The listing builds one solid part. Answer for the finished solid, in the listing's coordinates (mm). Give positions to 0.01 mm unless a question says otherwise; leave off trailing zeros. Order: outer loops, then holes, each group sorted by start corner. A loop starts at its lowest first (then second) coordinate and runs counter-clockwise, first axis right, second up.
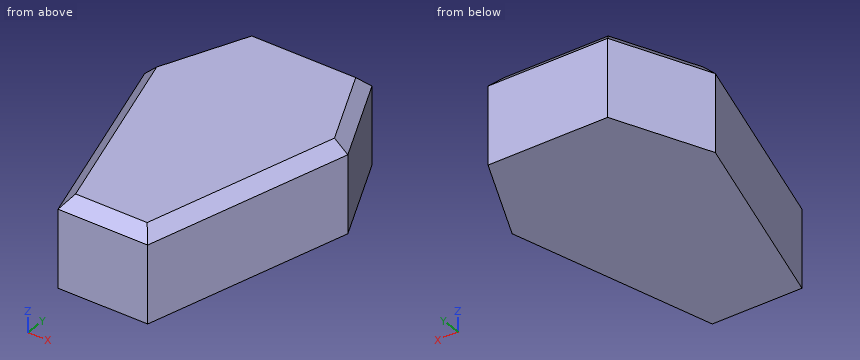
```python
from build123d import *

# Parameters (mm, degrees)
F1_DEPTH = 38.1
F2_SIZE  = 5.08
F3_T     = -7.62


with BuildPart() as f1:
    # F0 (on Top) → F1 (new body)
    with BuildSketch(Plane.XY):
        Polygon((17.9854446539, 64.1556447676), (-32.8145553461, 64.1556447676), (-50.5846425152, 24.8016563801), (-26.4645553461, -60.7637069099), (11.6354446539, -60.7637069099), (35.7555318229, 24.8016563801), align=None)
    extrude(amount=F1_DEPTH)

    # F2
    f2_edges = [f1.edges().sort_by_distance(p)[0] for p in [
        (-41.699599, 44.478651, 38.1),
        (-7.414555, 64.155645, 38.1),
        (26.870488, 44.478651, 38.1),
        (23.695488, -17.981025, 38.1),
        (-38.524599, -17.981025, 38.1),
        (-7.414555, -60.763707, 38.1),
    ]]
    chamfer(f2_edges, length=F2_SIZE)

    # F3 (hollow: no face is removed)
    offset(amount=F3_T, kind=Kind.INTERSECTION, mode=Mode.SUBTRACT)


solid = f1.part
```
1) Straight lines are drawn through the part: probe 1 along Z at (x, y) = (10, 4.5); probe 2 along Y at (x, z) = (-17, 24); probe 3 along X at (y, z) = (-48, 21.5). For each, find the intervals that lie inside material, in ascending order.
Geometry says:
probe 1: z = 0 to 7.62, 30.48 to 38.1
probe 2: y = -60.76 to -53.14, 56.54 to 64.16
probe 3: x = -30.06 to -22.15, 7.32 to 15.23
2) Find section A-A (x = -13). Write down the section's boundary in (y, z), then the cut area to 3 significant figures.
Geometry says:
outline: (-60.76, 0) - (64.16, 0) - (64.16, 33.02) - (59.08, 38.1) - (-55.68, 38.1) - (-60.76, 33.02) - close; hole (-53.14, 7.62) - (56.54, 7.62) - (56.54, 29.86) - (55.92, 30.48) - (-52.53, 30.48) - (-53.14, 29.86) - close
area: 2,230 mm2
3) Given P1, Ø10, axis at y = 2, z = 25.5, coming from the +X side; P2, Ø12, axis at y = -36, z = 26, coming from the -X side; P3, Ø10, axis at y = 15.5, z = 12.5, coming from the +X side, each flat-ended and moving along its own axis, determine where each tip first touches the part or whether it passes through.
Geometry says:
P1: stops at x = 30.74
P2: stops at x = -35.14
P3: stops at x = 34.54
4) Find section B-B (z = 22). Write down the section's boundary in (x, y).
Geometry says:
outline: (-50.58, 24.8) - (-26.46, -60.76) - (11.64, -60.76) - (35.76, 24.8) - (17.99, 64.16) - (-32.81, 64.16) - close; hole (-42.5, 24.2) - (-20.7, -53.14) - (5.87, -53.14) - (27.67, 24.2) - (13.07, 56.54) - (-27.89, 56.54) - close
5) Find section C-C (x = 9.5). Write down the section's boundary in (y, z).
Geometry says:
outline: (-60.76, 0) - (64.16, 0) - (64.16, 33.02) - (59.08, 38.1) - (-49.62, 38.1) - (-57.94, 35.84) - (-60.76, 33.02) - close; hole (-40.25, 7.62) - (56.54, 7.62) - (56.54, 29.86) - (55.92, 30.48) - (-37.98, 30.48) - (-40.25, 29.86) - close
